Part model, mm, in its own coordinate system. Round coordinates to 2 decimals unless told otherwise and drop trailing zeros. Write each loop counter-clockwise with the first axis right and the second up, starting at its lowest first coordinate (ties: lowest second). Pieces come first, ordered by that corner, then holes. Notation, with made-up numbers: (62.5, 23.25) -> (79.5, 23.25) arc R8 ccw to (79.5, 31.25) -> close; hole circle Ø11 at (-17.5, -14). An arc over 180 degrees is marked (long way). Return JSON: item names as keys, results as strings. Group by question number.
(1) Saw through at A-A (x = 0). List the corners of the cut face in (y, z), plus the area to 3 significant figures.
(2) Drop flat-ended pins along their axis: pin 1 Ø4 at (y, z) = (96, 9.5) entering from -X; pin 2 Ø3 at (y, z) = (-4.5, 17) entering from +X; pin 3 Ø8 at (x, z) = (16.5, 8) entering from +Y. Give the stop position or say it passes through.
(3) Drill centre lines: L1, parallel to X at y = 149.5, z = 14; L2, parallel to Y at x = 17.5, z = 6.25; L3, parallel to X at y = 146, z = 9.75. Where is each one in solid material? Low to high. Write a range as from..to.
(4) Saw through at B-B (z = 13). List the corners of the cut face in (x, y).
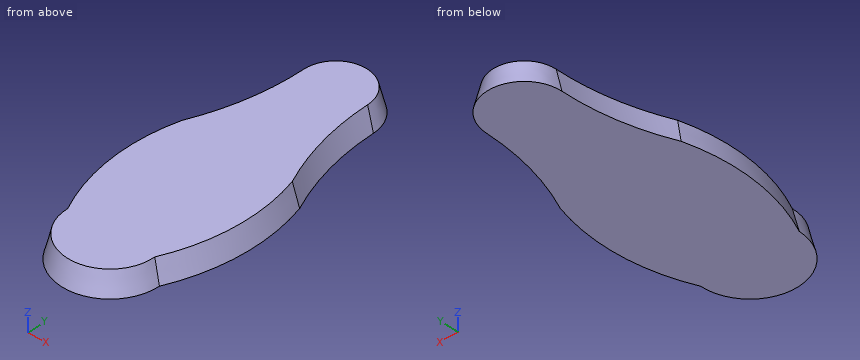
from build123d import *

# Parameters (mm, degrees)
BOSS_EXTRUDE1_DEPTH = 20
BOSS_EXTRUDE1_DRAFT = 14


with BuildPart() as part:
    # Sketch1 → Boss-Extrude1 (with draft: the straight prism first)
    with BuildSketch(Plane.XY):
        with BuildLine():
            ThreePointArc((-42.5, 0), (0, -42.5), (42.5, 0))
            ThreePointArc((42.5, 0), (58.212978051, 59.230104498), (52.040453066, 120.197332527))
            ThreePointArc((52.040453066, 120.197332527), (37.441607235, 164.047991362), (32.5, 210))
            ThreePointArc((32.5, 210), (0, 242.5), (-32.5, 210))
            ThreePointArc((-32.5, 210), (-37.441607235, 164.047991362), (-52.040453066, 120.197332527))
            ThreePointArc((-52.040453066, 120.197332527), (-58.212978051, 59.230104498), (-42.5, 0))
        make_face()
    extrude(amount=BOSS_EXTRUDE1_DEPTH)
    # Boss-Extrude1: the draft: its side faces are tilted about the plane it starts from
    boss_extrude1_sides = [part.faces().sort_by_distance(p)[0] for p in [
        (-58.212978051, 59.230104498, 10),
        (0, -42.5, 10),
        (58.212978051, 59.230104498, 10),
        (37.441607235, 164.047991362, 10),
        (0, 242.5, 10),
        (-37.441607235, 164.047991362, 10),
    ]]
    draft(boss_extrude1_sides, Plane.XY, BOSS_EXTRUDE1_DRAFT)


solid = part.part
Computed values:
{
 "1": {"outline": "(-42.5, 0) -> (242.5, 0) -> (237.51, 20) -> (-37.51, 20) -> close", "area": "5,600 mm2"},
 "2": {"pin 1": "x = -55.34", "pin 2": "x = 38.41", "pin 3": "y = 238.13"},
 "3": {"L1": "-37.51..37.51", "L2": "-37.01..235.52", "L3": "-39.65..39.65"},
 "4": {"outline": "(-48.99, 119.07) arc R167.8 ccw to (-39.25, 0.71) arc R39.26 ccw (long way) to (39.25, 0.71) arc R167.8 ccw to (48.99, 119.07) arc R219.37 cw to (29.26, 210) arc R29.26 ccw to (-29.26, 210) arc R219.37 cw to start"}
}
